```python
from build123d import *

# Parameters (mm, degrees)
EXTRUDE1_DEPTH     = 1.5875
MIRROR1_DEPTH      = 1.5875
CUT_EXTRUDE1_REACH = 534.229
SKETCH3_R          = 2.38125
CUT_EXTRUDE2_DEPTH = 533.229351555
FILLET1_R          = 25.4


# Read off the part's stored shape, not the designer's step: Mirror1
with BuildPart() as part:
    # Sketch1 → Extrude1 (new body)
    with BuildSketch(Plane(origin=(0, 0, 0), x_dir=(1, 0, 0), z_dir=(0, 1, 0))):
        Polygon((0, 0), (0, 158.75), (152.4, 311.15), (165.1, 311.15), (165.1, 234.95), (215.9, 234.95), (215.9, 0), align=None)
    extrude(amount=EXTRUDE1_DEPTH)

    # Mirror1 outline → Mirror1 (add)
    with BuildSketch(Plane(origin=(0, 0, 0), x_dir=(1, 0, 0), z_dir=(0, 1, 0))):
        Polygon((215.9, 0), (431.8, 0), (431.8, 158.75), (279.4, 311.15), (266.7, 311.15), (266.7, 234.95), (215.9, 234.95), align=None)
    extrude(amount=MIRROR1_DEPTH)

    # Sketch2 → Cut-Extrude1 (cut, up to next)
    with BuildSketch(Plane(origin=(0, 1.5875, 0), x_dir=(-1, 0, 0), z_dir=(0, 1, 0)), mode=Mode.PRIVATE) as cut_extrude1_sk1:
        Polygon((-276.225, -170.020724332), (-345.059, -170.020724332), (-345.059, -179.3875), (-377.825, -179.3875), (-377.825, -112.7125), (-345.059, -112.7125), (-345.059, -122.079275668), (-276.225, -122.079275668), align=None)
    cut_extrude1_tool1 = extrude(cut_extrude1_sk1.sketch, amount=-CUT_EXTRUDE1_REACH, mode=Mode.PRIVATE) & part.part
    add(cut_extrude1_tool1.solids().sort_by_distance((330.876817, 1.5875, -146.05))[0], mode=Mode.SUBTRACT)

    # Sketch3 → Cut-Extrude2 (cut, through all)
    with BuildSketch(Plane.XZ):
        with Locations(Location((400.05, -6.35, 0), (0, 0, 270))):
            Circle(SKETCH3_R)
        with Locations(Location((425.45, -146.05, 0), (0, 0, 270))):
            Circle(SKETCH3_R)
        with Locations(Location((355.710774635, -225.858969244, 0), (0, 0, 270))):
            Circle(SKETCH3_R)
        with Locations(Location((273.05, -304.8, 0), (0, 0, 270))):
            Circle(SKETCH3_R)
        with Locations(Location((273.05, -190.5, 0), (0, 0, 270))):
            Circle(SKETCH3_R)
        with Locations(Location((285.75, -6.35, 0), (0, 0, 270))):
            Circle(SKETCH3_R)
        with Locations(Location((158.75, -304.8, 0), (0, 0, 270))):
            Circle(SKETCH3_R)
        with Locations(Location((158.75, -155.575, 0), (0, 0, 270))):
            Circle(SKETCH3_R)
        with Locations(Location((146.05, -6.35, 0), (0, 0, 270))):
            Circle(SKETCH3_R)
        with Locations(Location((31.75, -6.35, 0), (0, 0, 270))):
            Circle(SKETCH3_R)
        with Locations(Location((6.35, -146.05, 0), (0, 0, 270))):
            Circle(SKETCH3_R)
        with Locations(Location((76.089225365, -225.858969244, 0), (0, 0, 270))):
            Circle(SKETCH3_R)
    extrude(amount=-CUT_EXTRUDE2_DEPTH, mode=Mode.SUBTRACT)

    # Fillet1
    fillet1_edges = [part.edges().sort_by_distance(p)[0] for p in [
        (0, 0.79375, -158.75),
        (431.8, 0.79375, -158.75),
    ]]
    fillet(fillet1_edges, radius=FILLET1_R)


solid = part.part
```
Input: part model. Units: mm. Frame: model coordinates. Round coordinates to 2 decimals unless told otherwise and drop trailing zeros. Loops run counter-clockwise (first coordinate to the right, second up) from the corner with the lowest first, then second, coordinate; pieces in that order, holes last.
1) Section query D-D on x = 124.5. Return the cut outline in (y, z).
Ans:
outline: (0, -283.25) - (1.59, -283.25) - (1.59, 0) - (0, 0) - close
2) Pin query (flat end, axial travel): pin 1 (0.8 mm diameter, centred on x = 360.5, y = 0.5, fed in from -Z); pin 2 (0.8 mm diameter, centred on y = 0.5, z = -287.5, fed in from +X). Return the tip coordinate at first contact, or that it passes through.
Ans:
pin 1: stops at z = -230.45
pin 2: stops at x = 303.45
3) Material intervals for line 1 (X direction, y = 1.15, z = -146.05) (3 decimals); line 2 (Z direction, x = 273.05, y = 0.6); line 3 (X direction, y = 0.35, z = -139) (3 decimals), sorted ascending.
Ans:
line 1: x = 0 to 3.969, 8.731 to 276.225, 377.825 to 423.069, 427.831 to 431.8
line 2: z = -311.15 to -307.18, -302.42 to -192.88, -188.12 to 0
line 3: x = 0 to 276.225, 377.825 to 431.8
4) Pull-direction query (Z, two-part tool) for faces 1 (the flat face through (78.91, 0.78, -237.66)), 2 (the flat face through (213, 0, -123)); classes: released by +Z, released by -Z, zero draft, split by the parting line, or undercut.
Ans:
face 1: released by -Z
face 2: zero draft
5) Section query B-B on z = -289.5. Return the cut outline in (x, y).
Ans:
outline: (130.75, 0) - (165.1, 0) - (165.1, 1.59) - (130.75, 1.59) - close; (266.7, 0) - (301.05, 0) - (301.05, 1.59) - (266.7, 1.59) - close
6) Section query C-C on y = 1.2. Count the separate pieces of the cut face and the enclosed holes in it, plus the area to 3 significant figures.
Ans:
separate pieces: 1
enclosed holes: 13
area: 97,700 mm2
7) Section query A-A on x = 369.5. Return the cut outline in (y, z).
Ans:
outline: (0, -221.05) - (1.59, -221.05) - (1.59, -179.39) - (0, -179.39) - close; (0, -112.71) - (1.59, -112.71) - (1.59, 0) - (0, 0) - close
